```python
from build123d import *

# Parameters (mm, degrees)
SKETCH2_R           = 3.5
BOSS_EXTRUDE1_DEPTH = 16
CHAMFER1_SIZE       = 0.25
SKETCH3_R           = 2.5
BOSS_EXTRUDE2_DEPTH = 38.4
CHAMFER2_SIZE       = 0.25
SKETCH4_R           = 6
BOSS_EXTRUDE3_DEPTH = 1


with BuildPart() as part:
    # Sketch2 → Boss-Extrude1 (new body)
    with BuildSketch(Plane(origin=(0, 0, 0), x_dir=(1, 0, 0), z_dir=(0, 1, 0))):
        with Locations(Location((0, 0, 0), (0, 0, 270))):
            Circle(SKETCH2_R)
    extrude(amount=BOSS_EXTRUDE1_DEPTH)

    # Chamfer1
    chamfer1_edges = [part.edges().sort_by_distance(p)[0] for p in [
        (0, 16, -3.5),
    ]]
    chamfer(chamfer1_edges, length=CHAMFER1_SIZE)

    # Sketch3 → Boss-Extrude2 (add)
    with BuildSketch(Plane.XZ):
        with Locations(Location((0, 0, 0), (0, 0, 90))):
            Circle(SKETCH3_R)
    extrude(amount=BOSS_EXTRUDE2_DEPTH)

    # Chamfer2
    chamfer2_edges = [part.edges().sort_by_distance(p)[0] for p in [
        (0, -38.4, -2.5),
    ]]
    chamfer(chamfer2_edges, length=CHAMFER2_SIZE)

    # Sketch4 → Boss-Extrude3 (add)
    with BuildSketch(Plane(origin=(0, 14, 0), x_dir=(1, 0, 0), z_dir=(0, 1, 0))):
        with Locations(Location((0, 0, 0), (0, 0, 270))):
            Circle(SKETCH4_R)
    extrude(amount=-BOSS_EXTRUDE3_DEPTH)


solid = part.part
```
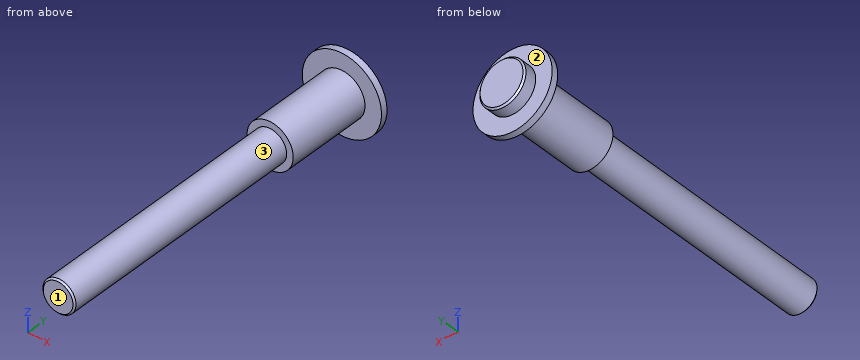
Input: part model. Units: mm. Frame: model coordinates. Face numbers are marked on the shaded views. A direction names the side the tool comes from. Coordinates: 2 decimals unless noted, no trailing zeros. Loops run counter-clockwise (first coordinate to the right, second up) from the corner with the lowest first, then second, coordinate; pieces in that order, holes last. Notation, with made-up numbers: (44, -6.5) -> (64, -6.5) arc R9 ccw to (64, 10.5) -> close; hole circle Ø7 at (27.5, 29). An arc over 180 degrees is marked (long way). Use a Markdown table: item, result.
1) Cut plane A-A (z = 0). Return the cut outline in (x, y), then the cut area to 3 significant figures.
Results found:
| item | result |
|---|---|
| outline | (-6, 13) -> (-3.5, 13) -> (-3.5, 0) -> (-2.5, 0) -> (-2.5, -38.15) -> (-2.25, -38.4) -> (2.25, -38.4) -> (2.5, -38.15) -> (2.5, 0) -> (3.5, 0) -> (3.5, 13) -> (6, 13) -> (6, 14) -> (3.5, 14) -> (3.5, 15.75) -> (3.25, 16) -> (-3.25, 16) -> (-3.5, 15.75) -> (-3.5, 14) -> (-6, 14) -> close |
| area | 309 mm2 |
2) Contact query for flat-ended pins moving along their axis: pin 1 (1.5 mm diameter, centred on x = -3, y = 2, fed in from +Z); pin 2 (4 mm diameter, centred on x = 3.5, z = 0.5, fed in from +Y); pin 3 (1.5 mm diameter, centred on y = 3, z = 0, fed in from +X); pin 4 (4 mm diameter, centred on x = -4, z = 2.5, fed in from -Y). Output: stop coordinate, or through.
Results found:
| item | result |
|---|---|
| pin 1 | stops at z = 2.68 |
| pin 2 | stops at y = 16 |
| pin 3 | stops at x = 3.5 |
| pin 4 | stops at y = 0 |
3) Cut plane B-B (x = 0). Return the cut outline in (y, z), then the cut area to 3 significant figures.
Results found:
| item | result |
|---|---|
| outline | (-38.4, -2.25) -> (-38.15, -2.5) -> (0, -2.5) -> (0, -3.5) -> (13, -3.5) -> (13, -6) -> (14, -6) -> (14, -3.5) -> (15.75, -3.5) -> (16, -3.25) -> (16, 3.25) -> (15.75, 3.5) -> (14, 3.5) -> (14, 6) -> (13, 6) -> (13, 3.5) -> (0, 3.5) -> (0, 2.5) -> (-38.15, 2.5) -> (-38.4, 2.25) -> close |
| area | 309 mm2 |
4) Material intervals for line 1 along Y through (x, z) = (-3, 3); line 2 along X through (y, z) = (14.5, -0.25); line 3 along Y through (x, z) = (1, 3), sorted ascending. Write a range as from..to.
Results found:
| item | result |
|---|---|
| line 1 | y = 13..14 |
| line 2 | x = -3.49..3.49 |
| line 3 | y = 0..16 |
5) Cut plane C-C (y = 8.5). Return the cut outline in (x, z), then the cut area to 3 significant figures.
Results found:
| item | result |
|---|---|
| outline | circle Ø7 at (0, 0) |
| area | 38.5 mm2 |
6) Cut plane D-D (x = 4.5). Return the cut outline in (y, z).
Results found:
| item | result |
|---|---|
| outline | (13, -3.97) -> (14, -3.97) -> (14, 3.97) -> (13, 3.97) -> close |
7) Access query for the marked faces 1, 2 and 3. Directions: +Z, -Z, +X, -X, +Y, -Y. A direction counts if a zero-diameter tool reaches every point of the face in a straight line with its end or side. Return the directions, or none.
Results found:
| item | result |
|---|---|
| face 1 | +Z, -Z, +X, -X, -Y |
| face 2 | +Y |
| face 3 | -Y |
